Could you check a few things on this model? Use its own coordinates, in mm. A direction names the side the tool comes from. Coordinates: 2 decimals unless noted, no trailing zeros. Loops run counter-clockwise (first coordinate to the right, second up) from the corner with the lowest first, then second, coordinate; pieces in that order, holes last. Notation, with made-up numbers: M 48,82 L 62,82 A33 ccw 62,114 Z; hole C 32.25,44.5 d8. An arc over 180 degrees is marked long. Write each question's results on one line, items separated by ' | '.
Autodesk Inventor part; units mm, degrees
ref_plane "YZ Plane" through (0, 0, 0) normal (1, 0, 0) x (0, 1, 0)
ref_plane "XZ Plane" through (0, 0, 0) normal (0, 1, 0) x (-1, 0, 0)
ref_plane "XY Plane" through (0, 0, 0) normal (0, 0, 1) x (1, 0, 0)
sketch "Sketch1" plane through (0, 0, 0) normal (0, 0, 1) x (1, 0, 0)
  line L0 (20, 0) -> (60, 0)
  line L1 (60, 0) -> (60, 70)
  line L2 (60, 70) -> (0, 70)
  line L3 (0, 70) -> (0, 55)
  line L4 (0, 55) -> (45, 55)
  line L5 (45, 55) -> (45, 15)
  line L6 (45, 15) -> (20, 15)
  line L7 (20, 15) -> (20, 0)
  point P0 (0, 0)
  dimension "d0" = 40
  dimension "d1" = 70
extrude "Extrusion1" add sketch "Sketch1" along normal blind 50
sketch "Sketch2" plane through (0, 70, 0) normal (0, 1, 0) x (1, 0, 0)
  line L0 (15, -15) -> (15, -35)
  line L1 (15, -35) -> (30, -35)
  line L2 (30, -35) -> (30, -15)
  line L3 (30, -15) -> (15, -15)
  point P0 (0, 0)
extrude "Extrusion2" cut sketch "Sketch2" against normal blind 15
sketch "Sketch3" plane through (60, 0, 0) normal (1, 0, 0) x (0, 0, -1)
  line L0 (-15, 25) -> (-35, 25)
  line L1 (-35, 25) -> (-35, 45)
  line L2 (-35, 45) -> (-15, 45)
  line L3 (-15, 45) -> (-15, 25)
  point P0 (0, 0)
extrude "Extrusion3" cut sketch "Sketch3" against normal blind 15
properties part number "P3-4"
(1) Imagine slicing it at C-C, the plane z = 16. List the corners of the cut face in (x, y) for me, and give its area (4 significant figures).
Reported:
outline: M 0,55 L 15,55 L 15,70 L 0,70 Z; M 20,0 L 60,0 L 60,25 L 45,25 L 45,15 L 20,15 Z; M 30,55 L 45,55 L 45,45 L 60,45 L 60,70 L 30,70 Z | area: 1,575 mm2
(2) Please list where these lines run through material, in increasing order: probe 1 along Y at (x, z) = (56, 19.5); probe 2 along Y at (x, z) = (31, 46.5); probe 3 along Z at (x, y) = (56, 27). Write a range as from..to.
Reported:
probe 1: y = 0..25, 45..70 | probe 2: y = 0..15, 55..70 | probe 3: z = 0..15, 35..50
(3) Imagine slicing it at B-B, the plane y = 64.5. List the corners of the cut face in (x, z) for me.
Reported:
outline: M 0,0 L 60,0 L 60,50 L 0,50 Z; hole M 15,15 L 30,15 L 30,35 L 15,35 Z
(4) If we mould it in two halves opening along X, with no side actions, what happens to faces 5 (the flat face through (0, 63, 25)), 6 (the flat face through (30.4, 70, 24.6)), 7 (the flat face through (23, 63, 15)), 8 (the flat face through (15, 63, 25))? For each: released by +X, released by -X, zero draft, split by the parting line, or undercut.
Reported:
face 5: released by -X | face 6: zero draft | face 7: undercut | face 8: undercut
(5) Imagine slicing it at D-D, the plane x = 54. List the corners of the cut face in (y, z) for me.
Reported:
outline: M 0,0 L 70,0 L 70,50 L 0,50 Z; hole M 25,15 L 45,15 L 45,35 L 25,35 Z
(6) Which directions (+Z, -Z, +X, -X, +Y, -Y) give clear straight access to the entire face, cutting with the end or side of a thin tool? Please do faces 1 (the flat face through (20, 8, 25)), 2 (the flat face through (33, 15, 25)), 3 (the flat face through (30, 63, 25)), 4 (the flat face through (53, 45, 25)).
Reported:
face 1: +Z, -Z, -X, -Y | face 2: +Z, -Z, -X | face 3: +Y | face 4: +X, -X
(7) Imagine slicing it at A-A, the plane x = 26. List the corners of the cut face in (y, z) for me, and give its area (3 significant figures).
Reported:
outline: M 0,0 L 15,0 L 15,50 L 0,50 Z; M 55,0 L 70,0 L 70,15 L 55,15 Z; M 55,35 L 70,35 L 70,50 L 55,50 Z | area: 1,200 mm2
(8) Will these pins go through, and if not, where does the flat tip stop? P1, Ø4.5, axis at y = 8, z = 25, coming from the -X side; P2, Ø20, axis at y = 40.5, z = 35, coming from the -X side.
Reported:
P1: stops at x = 20 | P2: stops at x = 45
